Design review of the part built by this model. Coordinates are the model's own, in mm. Face numbers are marked on the shaded views. Round coordinates to 2 decimals unless told otherwise and drop trailing zeros. Order: outer loops, then holes, each group sorted by start corner. A loop starts at its lowest first (then second) coordinate and runs counter-clockwise, first axis right, second up. Notation, with made-up numbers: (2, 31) - (43, 31) arc R3 ccw to (43, 35) - close; hole circle Ø7 at (52.25, 30.25). An arc over 180 degrees is marked (long way). Use CSV: the item, a comma, the result in double quotes.
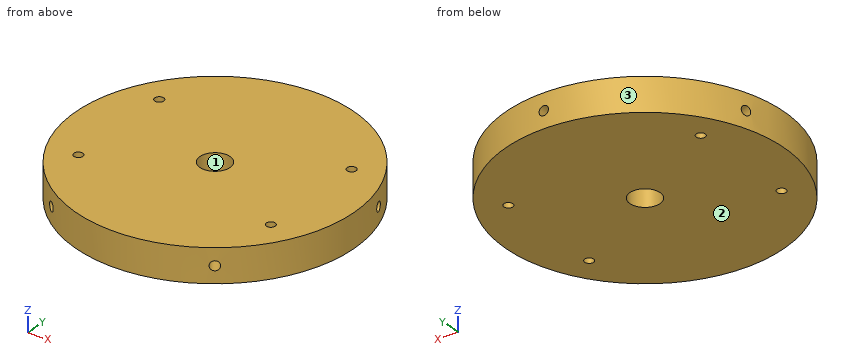
from build123d import *

# Parameters (mm, degrees)
SKETCH1_R                       = 62
BOSS_EXTRUDE1_DEPTH             = 15
F_4_0_4_DIAMETER_HOLE1_D        = 4
M12_CLEARANCE_HOLE1_D           = 13.5
M5_TAPPED_HOLE1_D               = 4.2
M5_TAPPED_HOLE1_DEPTH           = 12.4
M5_TAPPED_HOLE1_TIP             = 1.2618073
M5_TAPPED_HOLE1_ON_FACE_2_D     = 4.2
M5_TAPPED_HOLE1_ON_FACE_2_DEPTH = 12.4
M5_TAPPED_HOLE1_ON_FACE_2_TIP   = 1.2618073
M5_TAPPED_HOLE1_ON_FACE_3_D     = 4.2
M5_TAPPED_HOLE1_ON_FACE_3_DEPTH = 12.4
M5_TAPPED_HOLE1_ON_FACE_3_TIP   = 1.2618073
M5_TAPPED_HOLE1_ON_FACE_4_D     = 4.2
M5_TAPPED_HOLE1_ON_FACE_4_DEPTH = 12.4
M5_TAPPED_HOLE1_ON_FACE_4_TIP   = 1.2618073
M5_TAPPED_HOLE1_ON_FACE_5_D     = 4.2
M5_TAPPED_HOLE1_ON_FACE_5_DEPTH = 12.4
M5_TAPPED_HOLE1_ON_FACE_5_TIP   = 1.2618073


with BuildPart() as part:
    # Sketch1 → Boss-Extrude1 (new body)
    with BuildSketch(Plane.XY):
        Circle(SKETCH1_R)
    extrude(amount=BOSS_EXTRUDE1_DEPTH)

    # Ø4.0 (4) Diameter Hole1 (through all)
    with Locations(Plane(origin=(0, 0, 0), x_dir=(-1, 0, 0), z_dir=(0, 0, -1))):
        with Locations((-42.868257487, 24.75), (-42.868257487, -24.75), (42.868257487, -24.75), (42.868257487, 24.75)):
            Hole(F_4_0_4_DIAMETER_HOLE1_D / 2)

    # M12 Clearance Hole1 (through all)
    with Locations(Plane(origin=(0, 0, 0), x_dir=(-1, 0, 0), z_dir=(0, 0, -1))):
        with Locations((0, 0)):
            Hole(M12_CLEARANCE_HOLE1_D / 2)

    # M5 Tapped Hole1
    with Locations(Plane(origin=(0, 62, 7.5), x_dir=(1, 0, 0), z_dir=(0, 1, 0))):
        with Locations((0, 0)):
            Hole(M5_TAPPED_HOLE1_D / 2, depth=M5_TAPPED_HOLE1_DEPTH)
            with Locations((0, 0, -(M5_TAPPED_HOLE1_DEPTH + M5_TAPPED_HOLE1_TIP / 2))):  # 118° drill point
                Cone(0, M5_TAPPED_HOLE1_D / 2, M5_TAPPED_HOLE1_TIP, mode=Mode.SUBTRACT)

    # M5 Tapped Hole1 on face 2
    with Locations(Plane(origin=(58.96550401, 19.159053651, 7.5), x_dir=(-0.309016857306, 0.951056560832, 0), z_dir=(0.951056560832, 0.309016857306, 0))):
        with Locations((0, 0)):
            Hole(M5_TAPPED_HOLE1_ON_FACE_2_D / 2, depth=M5_TAPPED_HOLE1_ON_FACE_2_DEPTH)
            with Locations((0, 0, -(M5_TAPPED_HOLE1_ON_FACE_2_DEPTH + M5_TAPPED_HOLE1_ON_FACE_2_TIP / 2))):  # 118° drill point
                Cone(0, M5_TAPPED_HOLE1_ON_FACE_2_D / 2, M5_TAPPED_HOLE1_ON_FACE_2_TIP, mode=Mode.SUBTRACT)

    # M5 Tapped Hole1 on face 3
    with Locations(Plane(origin=(36.442685642, -50.159053651, 7.5), x_dir=(-0.809017116291, -0.58778508449, 0), z_dir=(0.58778508449, -0.809017116291, 0))):
        with Locations((0, 0)):
            Hole(M5_TAPPED_HOLE1_ON_FACE_3_D / 2, depth=M5_TAPPED_HOLE1_ON_FACE_3_DEPTH)
            with Locations((0, 0, -(M5_TAPPED_HOLE1_ON_FACE_3_DEPTH + M5_TAPPED_HOLE1_ON_FACE_3_TIP / 2))):  # 118° drill point
                Cone(0, M5_TAPPED_HOLE1_ON_FACE_3_D / 2, M5_TAPPED_HOLE1_ON_FACE_3_TIP, mode=Mode.SUBTRACT)

    # M5 Tapped Hole1 on face 4
    with Locations(Plane(origin=(-36.442685642, -50.159053651, 7.5), x_dir=(-0.809017116291, 0.58778508449, 0), z_dir=(-0.58778508449, -0.809017116291, 0))):
        with Locations((0, 0)):
            Hole(M5_TAPPED_HOLE1_ON_FACE_4_D / 2, depth=M5_TAPPED_HOLE1_ON_FACE_4_DEPTH)
            with Locations((0, 0, -(M5_TAPPED_HOLE1_ON_FACE_4_DEPTH + M5_TAPPED_HOLE1_ON_FACE_4_TIP / 2))):  # 118° drill point
                Cone(0, M5_TAPPED_HOLE1_ON_FACE_4_D / 2, M5_TAPPED_HOLE1_ON_FACE_4_TIP, mode=Mode.SUBTRACT)

    # M5 Tapped Hole1 on face 5
    with Locations(Plane(origin=(-58.96550401, 19.159053651, 7.5), x_dir=(-0.309016857306, -0.951056560832, 0), z_dir=(-0.951056560832, 0.309016857306, 0))):
        with Locations((0, 0)):
            Hole(M5_TAPPED_HOLE1_ON_FACE_5_D / 2, depth=M5_TAPPED_HOLE1_ON_FACE_5_DEPTH)
            with Locations((0, 0, -(M5_TAPPED_HOLE1_ON_FACE_5_DEPTH + M5_TAPPED_HOLE1_ON_FACE_5_TIP / 2))):  # 118° drill point
                Cone(0, M5_TAPPED_HOLE1_ON_FACE_5_D / 2, M5_TAPPED_HOLE1_ON_FACE_5_TIP, mode=Mode.SUBTRACT)


solid = part.part
1) To check wall thickness, follow L1, parallel to Y at x = 43, z = 7; L2, parallel to Y at x = -2.5, z = 6.75; L3, parallel to X at y = 4, z = 4.5. State the ranges of each line that lie inside material, in increasing order. Write a range as from..to.
Data:
L1,"y = -44.67..-26.75, -22.75..22.75, 26.75..44.67"
L2,"y = -61.95..-6.27, 6.27..61.95"
L3,"x = -61.87..-5.44, 5.44..61.87"
2) We need section C-C (y = 24.75). Give the boundary of the cut face in (x, z), then the cut area to 3 significant figures.
Data:
outline,"(-56.85, 0) - (-44.87, 0) - (-44.87, 15) - (-56.85, 15) - close; (-40.87, 0) - (40.87, 0) - (40.87, 15) - (-40.87, 15) - close; (44.87, 0) - (56.85, 0) - (56.85, 15) - (44.87, 15) - close"
area,"1,590 mm2"
3) Insertion check: pin 1 Ø4 at (x, z) = (-48.5, 5) entering from +Y; pin 2 Ø3.5 at (x, y) = (42.87, -24.75) entering from -Z; pin 3 Ø3.5 at (x, z) = (0, 7.5) entering from -Y; pin 4 Ø3 at (y, z) = (-10.5, 6.5) entering from -X. Each pin has a flat end and moves straight along its axis. Give the tip position at first contact, or say it passes through.
Data:
pin 1,"stops at y = 41.01"
pin 2,"passes through"
pin 3,"stops at y = -62"
pin 4,"stops at x = -61.34"
4) The part is to be moulded in two halves that separate along X. For the marked faces 1, 2 and 3, say which applies: +X half, -X half, draft (parallel to the pull), parting line (faces both ways), or undercut.
Data:
face 1,"undercut"
face 2,"draft"
face 3,"parting line"
5) We need section B-B (z = 11.5). Give the boundary of the cut face in (x, y).
Data:
outline,"circle Ø124 at (0, 0); hole circle Ø4 at (-42.87, -24.75); hole circle Ø4 at (-42.87, 24.75); hole circle Ø13.5 at (0, 0); hole circle Ø4 at (42.87, -24.75); hole circle Ø4 at (42.87, 24.75)"
6) We need section A-A (y = 0). Give the boundary of the cut face in (x, z), then the cut area to 3 significant figures.
Data:
outline,"(-62, 0) - (-6.75, 0) - (-6.75, 15) - (-62, 15) - close; (6.75, 0) - (62, 0) - (62, 15) - (6.75, 15) - close"
area,"1,660 mm2"
